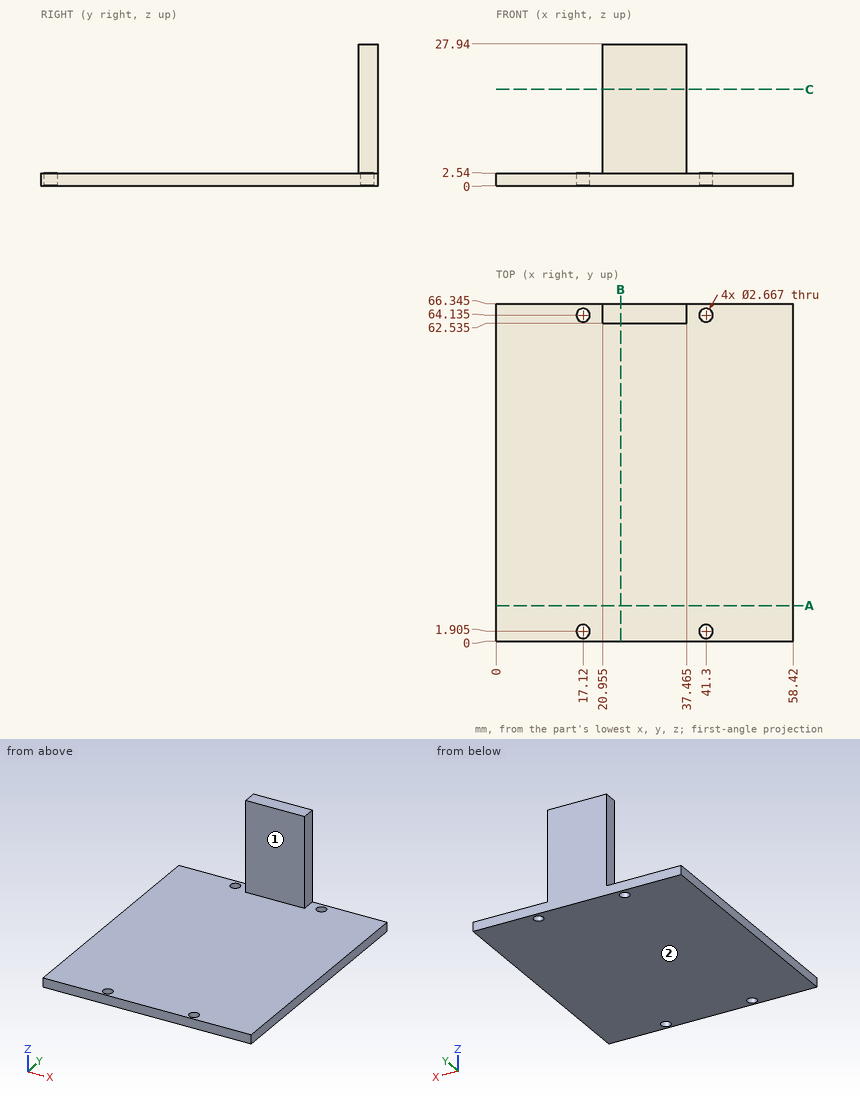
Job drawing, mm, ordinate dimensions from the low corner. One solid piece. A direction names the side the tool comes from. Give positions to 0.01 mm unless a question says otherwise; leave off trailing zeros. Order: outer loops, then holes, each group sorted by start corner. A loop starts at its lowest first (then second) coordinate and runs counter-clockwise, first axis right, second up. Notation, with made-up numbers: (53, -13.5) - (82, -13.5) arc R11 ccw to (82, -8.5) - close; hole circle Ø4 at (-4.5, 71). An arc over 180 degrees is marked (long way). Answer in a Markdown table with one row per item.
1. Probe probe 1 along Z at (x, y) = (47, 22.5); probe 2 along Y at (x, z) = (29.5, 18.5) (1 decimal). List the from-to ranges inside material, lowest first. Write a range as [from, to].
Data:
| item | result |
|---|---|
| probe 1 | z = [0, 2.54] |
| probe 2 | y = [62.5, 66.3] |
2. Saw through at A-A, the plane y = 7. Give the cut face in (x, z), plus the area to 3 significant figures.
Data:
| item | result |
|---|---|
| outline | (0, 0) - (58.42, 0) - (58.42, 2.54) - (0, 2.54) - close |
| area | 148 mm² |
3. Saw through at C-C, the plane z = 19. Give the cut face in (x, y) (1 decimal).
Data:
| item | result |
|---|---|
| outline | (21, 62.5) - (37.5, 62.5) - (37.5, 66.3) - (21, 66.3) - close |
4. Saw through at B-B, the plane x = 24.5. Give the cut face in (y, z) (1 decimal), plus the area to 3 significant figures.
Data:
| item | result |
|---|---|
| outline | (0, 0) - (66.3, 0) - (66.3, 27.9) - (62.5, 27.9) - (62.5, 2.5) - (0, 2.5) - close |
| area | 265 mm² |
5. Tool access for the marked faces 1 and 2: list every direction of +Z, -Z, +X, -X, +Y, -Y with a clear straight run to the whole face (end or side of a thin tool).
Data:
| item | result |
|---|---|
| face 1 | +Z, +X, -X, -Y |
| face 2 | -Z, +X, -X, +Y, -Y |
6. Flat gauge pins, fed straight in: pin 1 (2 mm diameter, centred on x = 36.5, y = 18.5, fed in from +Z); pin 2 (1.1 mm diameter, centred on y = 65, z = 16, fed in from +X) (3 decimals); pin 3 (2 mm diameter, centred on x = 41.3, y = 64.14, fed in from +Z); pin 4 (12 mm diameter, centred on x = 38, z = 21, fed in from -Y) (1 decimal). Where does each tip first touch, or does it go through?
Data:
| item | result |
|---|---|
| pin 1 | stops at z = 2.54 |
| pin 2 | stops at x = 37.465 |
| pin 3 | passes through |
| pin 4 | stops at y = 62.5 |
